Geometry: final body of the model. Coordinates: model frame, mm. A direction names the side the tool comes from. Give positions to 0.01 mm unless a question says otherwise; leave off trailing zeros. Write each loop counter-clockwise with the first axis right and the second up, starting at its lowest first coordinate (ties: lowest second). Pieces come first, ordered by that corner, then holes. Notation, with made-up numbers: M -12.5,18.25 L 34.5,18.25 A19 ccw 34.5,51.25 Z; hole C 28.5,63 d5. An arc over 180 degrees is marked long. Use a Markdown table: item, result. Add a question column.
(1) Cut plane B-B (x = 37.5). Output: boundary loops of the cut face in (y, z), plus the area to 3 significant figures.
(2) Cut plane C-C (x = 16.6). Output: boundary loops of the cut face in (y, z).
(3) Draft query along X for faces 3 (the flat face through (-1, 2, -1)), 4 (the cylindrical face through (37.4, 1, -39.9)). Return one class per face: released by +X, released by -X, zero draft, split by the parting line, or undercut.
(4) Cut plane A-A (z = 45). Output: boundary loops of the cut face in (x, y), plus the area to 3 significant figures.
(5) Material intervals for L1, parallel to X at y = 0.95, z = -22.5; L2, parallel to Z at x = -37.5, y = 1.6; L3, parallel to X at y = 1.35, z = 45, sorted ascending.
(6) Reachability of faces 1 (the cylindrical face through (37.6, 1, -50.1)), 2 (the flat face through (-1, 0, -1)) from +Z, -Z, +X, -X, +Y, -Y: full face, straight path, thin tool, end or side. Return the list, or none.
(7) Cut plane D-D (y = 1.6). Output: boundary loops of the cut face in (x, z), plus the area to 3 significant figures.
(8) Pin query (flat end, axial travel): pin 1 Ø3 at (x, z) = (-37.5, 45) entering from +Y (1 decimal). Return the tip coordinate at first contact, or that it passes through.
```python
from build123d import *

# Parameters (mm, degrees)
SKETCH1_W           = 95
SKETCH1_H           = 115
SKETCH1_R           = 2.6
BOSS_EXTRUDE1_DEPTH = 2
CUT_EXTRUDE1_DEPTH  = 75.608980693
FILLET1_R           = 1.5
CUT_EXTRUDE2_DEPTH  = 75.608980693


with BuildPart() as part:
    # Sketch1 → Boss-Extrude1 (new body)
    with BuildSketch(Plane(origin=(0, 0, 0), x_dir=(1, 0, 0), z_dir=(0, 1, 0))):
        Rectangle(SKETCH1_W, SKETCH1_H)
        with Locations(Location((-37.5, 45, 0), (0, 0, 270))):
            Circle(SKETCH1_R, mode=Mode.SUBTRACT)
        with Locations(Location((37.5, 45, 0), (0, 0, 90))):
            Circle(SKETCH1_R, mode=Mode.SUBTRACT)
        with Locations(Location((37.5, -45, 0), (0, 0, 270))):
            Circle(SKETCH1_R, mode=Mode.SUBTRACT)
        with Locations(Location((-37.5, -45, 0), (0, 0, 90))):
            Circle(SKETCH1_R, mode=Mode.SUBTRACT)
    extrude(amount=BOSS_EXTRUDE1_DEPTH)

    # Sketch2 → Cut-Extrude1 (cut, through all)
    with BuildSketch(Plane(origin=(0, 2, 0), x_dir=(1, 0, 0), z_dir=(0, 1, 0))):
        with BuildLine():
            Line((-34.9, 47.5), (-34.9, 42.5))
            ThreePointArc((-34.9, 42.5), (-37.5, 39.9), (-40.1, 42.5))
            Line((-40.1, 42.5), (-40.1, 47.5))
            ThreePointArc((-40.1, 47.5), (-37.5, 50.1), (-34.9, 47.5))
        make_face()
        with BuildLine():
            Line((34.9, 47.5), (34.9, 42.5))
            ThreePointArc((34.9, 42.5), (37.5, 39.9), (40.1, 42.5))
            Line((40.1, 42.5), (40.1, 47.5))
            ThreePointArc((40.1, 47.5), (37.5, 50.1), (34.9, 47.5))
        make_face()
    extrude(amount=-CUT_EXTRUDE1_DEPTH, mode=Mode.SUBTRACT)

    # Fillet1
    fillet1_edges = [part.edges().sort_by_distance(p)[0] for p in [
        (47.5, 1, 57.5),
        (-47.5, 1, 57.5),
        (-47.5, 1, -57.5),
        (47.5, 1, -57.5),
    ]]
    fillet(fillet1_edges, radius=FILLET1_R)

    # Sketch3 → Cut-Extrude2 (cut, through all)
    with BuildSketch(Plane.XZ):
        with BuildLine():
            Line((15, -37.5), (15, -12.5))
            ThreePointArc((15, -12.5), (16.6, -10.9), (18.2, -12.5))
            Line((18.2, -12.5), (18.2, -37.5))
            ThreePointArc((18.2, -37.5), (16.6, -39.1), (15, -37.5))
        make_face()
        with BuildLine():
            Line((-15, -37.5), (-15, -12.5))
            ThreePointArc((-15, -12.5), (-16.6, -10.9), (-18.2, -12.5))
            Line((-18.2, -12.5), (-18.2, -37.5))
            ThreePointArc((-18.2, -37.5), (-16.6, -39.1), (-15, -37.5))
        make_face()
    extrude(amount=-CUT_EXTRUDE2_DEPTH, mode=Mode.SUBTRACT)


solid = part.part
```
Answer list:
| question | item | result |
|---|---|---|
| 1 | outline | M 0,-57.5 L 2,-57.5 L 2,-50.1 L 0,-50.1 Z; M 0,-39.9 L 2,-39.9 L 2,42.4 L 0,42.4 Z; M 0,47.6 L 2,47.6 L 2,57.5 L 0,57.5 Z |
| 1 | area | 199 mm² |
| 2 | outline | M 0,-57.5 L 2,-57.5 L 2,-39.1 L 0,-39.1 Z; M 0,-10.9 L 2,-10.9 L 2,57.5 L 0,57.5 Z |
| 3 | face 3 | zero draft |
| 3 | face 4 | undercut |
| 4 | outline | M -47.5,0 L -40.1,0 L -40.1,2 L -47.5,2 Z; M -34.9,0 L 34.9,0 L 34.9,2 L -34.9,2 Z; M 40.1,0 L 47.5,0 L 47.5,2 L 40.1,2 Z |
| 4 | area | 169 mm² |
| 5 | L1 | -47.5 to -18.2, -15 to 15, 18.2 to 47.5 |
| 5 | L2 | -57.5 to -50.1, -39.9 to 42.4, 47.6 to 57.5 |
| 5 | L3 | -47.5 to -40.1, -34.9 to 34.9, 40.1 to 47.5 |
| 6 | face 1 | +Y, -Y |
| 6 | face 2 | +Z, -Z, +X, -X, -Y |
| 7 | outline | M -47.5,-56 A1.5 ccw -46,-57.5 L 46,-57.5 A1.5 ccw 47.5,-56 L 47.5,56 A1.5 ccw 46,57.5 L -46,57.5 A1.5 ccw -47.5,56 Z; hole M -40.1,-47.5 A2.6 ccw -34.9,-47.5 L -34.9,-42.5 A2.6 ccw -40.1,-42.5 Z; hole C -37.5,45 d5.2; hole M -18.2,-37.5 A1.6 ccw -15,-37.5 L -15,-12.5 A1.6 ccw -18.2,-12.5 Z; hole M 15,-37.5 A1.6 ccw 18.2,-37.5 L 18.2,-12.5 A1.6 ccw 15,-12.5 Z; hole M 34.9,-47.5 A2.6 ccw 40.1,-47.5 L 40.1,-42.5 A2.6 ccw 34.9,-42.5 Z; hole C 37.5,45 d5.2 |
| 7 | area | 10,600 mm² |
| 8 | pin 1 | through |
